```python
from build123d import *

# Parameters (mm, degrees)
CYLINDER006_R          = 25
CYLINDER006_DEPTH      = 3
CYLINDER006_ROLL_ANGLE = 90
CYLINDER003_R          = 5
CYLINDER003_DEPTH      = 11
CYLINDER003_ROLL_ANGLE = 90
CYLINDER005_R          = 30
CYLINDER005_DEPTH      = 3
CYLINDER005_ROLL_ANGLE = 90
CYLINDER004_R          = 15
CYLINDER004_DEPTH      = 4
CYLINDER004_ROLL_ANGLE = 90
CYLINDER002_R          = 4
CYLINDER002_DEPTH      = 32
CYLINDER002_ROLL_ANGLE = 90


with BuildPart() as bein004:
    # Cylinder006 → Cylinder006 (new body)
    with BuildSketch(Plane.XY):
        Circle(CYLINDER006_R)
    extrude(amount=CYLINDER006_DEPTH)


with BuildPart() as bein004_1:
    # Cylinder006 roll: moved
    add(bein004.part.rotate(Axis((0, 0, 0), (1, 0, 0)), CYLINDER006_ROLL_ANGLE))


with BuildPart() as bein004_2:
    # Cylinder006 placement: moved
    add(bein004_1.part.moved(Location((32, 3, 35.5))))


with BuildPart() as bein001:
    # Cylinder003 → Cylinder003 (new body)
    with BuildSketch(Plane.XY):
        Circle(CYLINDER003_R)
    extrude(amount=CYLINDER003_DEPTH)


with BuildPart() as bein001_1:
    # Cylinder003 roll: moved
    add(bein001.part.rotate(Axis((0, 0, 0), (1, 0, 0)), CYLINDER003_ROLL_ANGLE))


with BuildPart() as bein001_2:
    # Cylinder003 placement: moved
    add(bein001_1.part.moved(Location((32, 12, 35.5))))


with BuildPart() as bein003:
    # Cylinder005 → Cylinder005 (new body)
    with BuildSketch(Plane.XY):
        Circle(CYLINDER005_R)
    extrude(amount=CYLINDER005_DEPTH)


with BuildPart() as bein003_1:
    # Cylinder005 roll: moved
    add(bein003.part.rotate(Axis((0, 0, 0), (1, 0, 0)), CYLINDER005_ROLL_ANGLE))


with BuildPart() as bein003_2:
    # Cylinder005 placement: moved
    add(bein003_1.part.moved(Location((32, 5, 35.5))))


with BuildPart() as bein002:
    # Cylinder004 → Cylinder004 (new body)
    with BuildSketch(Plane.XY):
        Circle(CYLINDER004_R)
    extrude(amount=CYLINDER004_DEPTH)


with BuildPart() as bein002_1:
    # Cylinder004 roll: moved
    add(bein002.part.rotate(Axis((0, 0, 0), (1, 0, 0)), CYLINDER004_ROLL_ANGLE))


with BuildPart() as bein002_2:
    # Cylinder004 placement: moved
    add(bein002_1.part.moved(Location((32, 7, 35.5))))


with BuildPart() as cut002:
    # Cylinder002 → Cylinder002 (new body)
    with BuildSketch(Plane.XY):
        Circle(CYLINDER002_R)
    extrude(amount=CYLINDER002_DEPTH)


with BuildPart() as cut002_1:
    # Cylinder002 roll: moved
    add(cut002.part.rotate(Axis((0, 0, 0), (1, 0, 0)), CYLINDER002_ROLL_ANGLE))


with BuildPart() as cut002_2:
    # Cylinder002 placement: moved
    add(cut002_1.part.moved(Location((32, 34, 35.5))))

    # Fusion002: union bein001, bein003, bein002
    add(bein001_2.part)
    add(bein003_2.part)
    add(bein002_2.part)

    # Cut002: cut bein004
    add(bein004_2.part, mode=Mode.SUBTRACT)


solid = cut002_2.part
```
Verification items for the finished model (mm, model axes). A direction names the side the tool comes from. Give positions to 0.01 mm unless a question says otherwise; leave off trailing zeros. Loops run counter-clockwise (first coordinate to the right, second up) from the corner with the lowest first, then second, coordinate; pieces in that order, holes last.
1. Go/stop test with flat-tipped pins: pin 1 Ø25 at (x, z) = (27, 31) entering from -Y; pin 2 Ø8 at (y, z) = (8, 55.5) entering from -X; pin 3 Ø8 at (x, z) = (14.5, 22.5) entering from +Y; pin 4 Ø12 at (x, y) = (42.5, 26.5) entering from +Z. Record where each tip stops, or that it passes through.
2. Section check C-C, the plane y = 18.5. Enter the section's corners in (x, z), then the cut area to 3 significant figures.
3. Section check B-B, the plane x = 32. Enter the section's corners in (y, z).
4. Section check A-A, the plane z = 35.5. Enter the section's corners in (x, y).
5. Thickness scan on line 1 (Z direction, x = 32, y = 2.6); line 2 (Y direction, x = 21, z = 25); line 3 (Y direction, x = 42, z = 27). Record the ranges inside material, lowest first.
6. Mould release check, pull along Z, two halves, no side actions. Record for faces 1 (the flat face through (32, 3, 36)), 2 (the flat face through (18, 5, 29)), 3 (the cylindrical face through (12.16, 2.51, 20.29)), 4 (the cylindrical face through (27.005, 9.535, 35.72)): released by +Z, released by -Z, zero draft, split by the parting line, or undercut.
7. Set-up check for faces 5 (the cylindrical face through (8.19, 3.52, 17.25)), 6 (the cylindrical face through (20.944, 6.014, 45.638)): record each of +Z, -Z, +X, -X, +Y, -Y from which the full face is reachable in a straight line by a thin tool's end or side.
8. Section check D-D, the plane x = 21. Enter the section's corners in (y, z), then the cut area to 3 significant figures.
Geometry says:
1. pin 1: stops at y = 3
1. pin 2: stops at x = 7.53
1. pin 3: stops at y = 5
1. pin 4: passes through
2. outline: circle Ø8 at (32, 35.5)
2. area: 50.3 mm2
3. outline: (2, 5.5) - (5, 5.5) - (5, 20.5) - (7, 20.5) - (7, 30.5) - (12, 30.5) - (12, 31.5) - (34, 31.5) - (34, 39.5) - (12, 39.5) - (12, 40.5) - (7, 40.5) - (7, 50.5) - (5, 50.5) - (5, 65.5) - (2, 65.5) - (2, 60.5) - (3, 60.5) - (3, 10.5) - (2, 10.5) - close
4. outline: (2, 2) - (7, 2) - (7, 3) - (57, 3) - (57, 2) - (62, 2) - (62, 5) - (47, 5) - (47, 7) - (37, 7) - (37, 12) - (36, 12) - (36, 34) - (28, 34) - (28, 12) - (27, 12) - (27, 7) - (17, 7) - (17, 5) - (2, 5) - close
5. line 1: z = 5.5 to 10.5, 60.5 to 65.5
5. line 2: y = 3 to 5
5. line 3: y = 3 to 7
6. face 1: undercut
6. face 2: zero draft
6. face 3: undercut
6. face 4: split by the parting line
7. face 5: +Y, -Y
7. face 6: +Y
8. outline: (2, 7.59) - (5, 7.59) - (5, 25.3) - (7, 25.3) - (7, 45.7) - (5, 45.7) - (5, 63.41) - (2, 63.41) - (2, 57.95) - (3, 57.95) - (3, 13.05) - (2, 13.05) - close
8. area: 163 mm2
